```python
from build123d import *

# Parameters (mm, degrees)
F0_W     = 100
F0_H     = 65
F1_DEPTH = 50
F2_R     = 5
F3_T     = -2.5


with BuildPart() as f1:
    # F0 (on Front) → F1 (new body)
    with BuildSketch(Plane.XZ):
        Rectangle(F0_W, F0_H)
    extrude(amount=F1_DEPTH)

    # F2
    f2_edges = [f1.edges().sort_by_distance(p)[0] for p in [
        (-50, -25, 32.5),
        (-50, -25, -32.5),
        (50, -25, 32.5),
        (50, -25, -32.5),
    ]]
    fillet(f2_edges, radius=F2_R)

    # F3
    f3_openings = [f1.faces().sort_by_distance(p)[0] for p in [
        (0, -50, 0),
        (0, 0, 0),
    ]]
    offset(amount=F3_T, openings=f3_openings)


solid = f1.part
```
Verification items for the finished model (mm, model axes). A direction names the side the tool comes from. Round coordinates to 2 decimals unless told otherwise and drop trailing zeros. Write each loop counter-clockwise with the first axis right and the second up, starting at its lowest first coordinate (ties: lowest second). Pieces come first, ordered by that corner, then holes.
1. Section check B-B on x = 36. Enter the section's corners in (y, z).
2. Section check A-A on z = -6. Enter the section's corners in (x, y), plus the area to 3 significant figures.
3. Section check C-C on y = -45. Enter the section's corners in (x, z), plus the area to 3 significant figures.
4. Scan lines: L1, parallel to X at y = -33.5, z = 16.5; L2, parallel to Z at x = -37, y = -8; L3, parallel to X at y = -16, z = 29.5. Record each from-to range of solid material in increasing order.
5. Access from +Z, -Z, +X, -X, +Y, -Y to the whole of each face (thin tool, end or side, straight path). Record for faces 4 (the flat face through (-47.5, -25, 0)), 5 (the cylindrical face through (48.57, -25.35, 31)).
6. Draft check along Z on faces 1 (the flat face through (-1, -25, 32.5)), 2 (the cylindrical face through (47, -25, -29)), 3 (the flat face through (50, -25, 0)). Enter one of: +Z half, -Z half, draft (parallel to the pull), parting line (faces both ways), or undercut.
Answer:
1. outline: (-50, -32.5) - (0, -32.5) - (0, -30) - (-50, -30) - close; (-50, 30) - (0, 30) - (0, 32.5) - (-50, 32.5) - close
2. outline: (-50, -50) - (-47.5, -50) - (-47.5, 0) - (-50, 0) - close; (47.5, -50) - (50, -50) - (50, 0) - (47.5, 0) - close
2. area: 250 mm2
3. outline: (-50, -27.5) arc R5 ccw to (-45, -32.5) - (45, -32.5) arc R5 ccw to (50, -27.5) - (50, 27.5) arc R5 ccw to (45, 32.5) - (-45, 32.5) arc R5 ccw to (-50, 27.5) - close; hole (-47.5, -27.5) arc R2.5 ccw to (-45, -30) - (45, -30) arc R2.5 ccw to (47.5, -27.5) - (47.5, 27.5) arc R2.5 ccw to (45, 30) - (-45, 30) arc R2.5 ccw to (-47.5, 27.5) - close
3. area: 784 mm2
4. L1: x = -50 to -47.5, 47.5 to 50
4. L2: z = -32.5 to -30, 30 to 32.5
4. L3: x = -49.58 to -46.5, 46.5 to 49.58
5. face 4: +Y, -Y
5. face 5: +Z, +X, +Y, -Y
6. face 1: +Z half
6. face 2: undercut
6. face 3: draft
